For this review, take the finished solid that the model builds, in its own axes (mm). A direction names the side the tool comes from. Round coordinates to 2 decimals unless told otherwise and drop trailing zeros. Write each loop counter-clockwise with the first axis right and the second up, starting at its lowest first coordinate (ties: lowest second). Pieces come first, ordered by that corner, then holes. Notation, with made-up numbers: M 76,82 L 131,82 A18 cw 131,94 Z; hole C -30.75,37.25 d4. An arc over 180 degrees is marked long. One line per question, with ' | ' between items.
```python
from build123d import *

# Parameters (mm, degrees)
BOSS_EXTRUDE1_DEPTH     = 76.2
F_1_4_CLEARANCE_HOLE1_D = 7.14248


with BuildPart() as part:
    # Sketch2 → Boss-Extrude1 (new body)
    with BuildSketch(Plane.XY):
        Polygon((-19.05, 15.875), (-22.225, 15.875), (-22.225, -15.875), (22.225, -15.875), (22.225, 15.875), (19.05, 15.875), (19.05, -12.7), (-19.05, -12.7), align=None)
    extrude(amount=BOSS_EXTRUDE1_DEPTH)

    # 1/4 Clearance Hole1 (through all)
    with Locations(Plane(origin=(22.225, 0, 0), x_dir=(0, 0, -1), z_dir=(1, 0, 0))):
        with Locations((-19.05, 0), (-63.5, 0)):
            Hole(F_1_4_CLEARANCE_HOLE1_D / 2)


solid = part.part
```
Item 1: Take a section at D-D (x = 1). Write out the cut boundary in (y, z) (3 decimals).
Results:
outline: M -15.875,0 L -12.7,0 L -12.7,76.2 L -15.875,76.2 Z
Item 2: Machinability: for faces 1 (the face through (22.225, 0, 38)), 2 (the face through (0, -12.7, 38)), which of the approach directions +Z, -Z, +X, -X, +Y, -Y give a long, thin tool a straight path to every point of the face, cutting with its end or side? Answer none if there is none.
Results:
face 1: +Z, -Z, +X, +Y, -Y | face 2: +Z, -Z, +Y
Item 3: Take a section at B-B (z = 63.5). Write out the cut boundary in (x, y) (3 decimals), then the cut area to 3 significant figures.
Results:
outline: M -22.225,-15.875 L 22.225,-15.875 L 22.225,-3.571 L 19.05,-3.571 L 19.05,-12.7 L -19.05,-12.7 L -19.05,-3.571 L -22.225,-3.571 Z; M -22.225,3.571 L -19.05,3.571 L -19.05,15.875 L -22.225,15.875 Z; M 19.05,3.571 L 22.225,3.571 L 22.225,15.875 L 19.05,15.875 Z | area: 277 mm2
Item 4: Mouldability with a two-part tool opening along Y and no side actions: class faces 3 (the face through (21, 15.875, 38)), 4 (the face through (19.05, 2, 38)), 5 (the face through (20.62, -1.37, 66.8)) as +Y half, -Y half, draft (parallel to the pull), parting line (faces both ways), or undercut.
Results:
face 3: +Y half | face 4: draft | face 5: undercut
Item 5: Insertion check: pin 1 Ø5.5 at (y, z) = (0, 63.5) entering from -X; pin 2 Ø12 at (x, z) = (10, 13.5) entering from +Y; pin 3 Ø11.5 at (y, z) = (0, 63.5) entering from -X (3 decimals). Each pin has a flat end and moves straight along its axis. Give the tip position at first contact, or say it passes through.
Results:
pin 1: through | pin 2: y = -12.7 | pin 3: x = -22.225
Item 6: Take a section at A-A (y = 0). Write out the cut boundary in (x, z) (3 decimals), then the cut area to 3 significant figures.
Results:
outline: M -22.225,0 L -19.05,0 L -19.05,15.479 L -22.225,15.479 Z; M -22.225,22.621 L -19.05,22.621 L -19.05,59.929 L -22.225,59.929 Z; M -22.225,67.071 L -19.05,67.071 L -19.05,76.2 L -22.225,76.2 Z; M 19.05,0 L 22.225,0 L 22.225,15.479 L 19.05,15.479 Z; M 19.05,22.621 L 22.225,22.621 L 22.225,59.929 L 19.05,59.929 Z; M 19.05,67.071 L 22.225,67.071 L 22.225,76.2 L 19.05,76.2 Z | area: 393 mm2
Item 7: Take a section at C-C (y = 11.5). Write out the cut boundary in (x, z) (3 decimals), then the cut area to 3 significant figures.
Results:
outline: M -22.225,0 L -19.05,0 L -19.05,76.2 L -22.225,76.2 Z; M 19.05,0 L 22.225,0 L 22.225,76.2 L 19.05,76.2 Z | area: 484 mm2
Item 8: To check wall thickness, follow line 1 along X through (y, z) = (-4, 16) (3 decimals); line 2 along Y through (x, z) = (20, 19) (3 decimals); line 3 along Y through (x, z) = (15.5, 14.5) (3 decimals). State the ranges of each line that lie inside material, in increasing order. Write a range as from..to.
Results:
line 1: -22.225..-19.05, 19.05..22.225 | line 2: -15.875..-3.571, 3.571..15.875 | line 3: -15.875..-12.7
